from build123d import *

# Parameters (mm, degrees)
SKETCH2_R           = 1.7
BOSS_EXTRUDE1_DEPTH = 3.175
CUT_EXTRUDE1_DEPTH  = 4.175


with BuildPart() as part:
    # Sketch2 → Boss-Extrude1 (new body)
    with BuildSketch(Plane.XY):
        with BuildLine():
            Line((54.582717937, -59.58290593), (54.582717937, 171.394622999))
            ThreePointArc((54.582717937, 171.394622999), (24.582717937, 201.394622999), (-5.417282063, 171.394622999))
            Line((-5.417282063, 171.394622999), (-5.417282063, -59.58290593))
            ThreePointArc((-5.417282063, -59.58290593), (24.582717937, -89.58290593), (54.582717937, -59.58290593))
        make_face()
        with Locations((27.882717937, 197.940291196)):
            Circle(SKETCH2_R, mode=Mode.SUBTRACT)
        with Locations((-2.167282063, -59.58290593)):
            Circle(SKETCH2_R, mode=Mode.SUBTRACT)
        with Locations((5.667611541, -78.498012327)):
            Circle(SKETCH2_R, mode=Mode.SUBTRACT)
        with Locations((21.182717937, -86.115951364)):
            Circle(SKETCH2_R, mode=Mode.SUBTRACT)
        with Locations((51.332717937, 171.394622999)):
            Circle(SKETCH2_R, mode=Mode.SUBTRACT)
        with Locations((-2.167282063, 59.305858535)):
            Circle(SKETCH2_R, mode=Mode.SUBTRACT)
        with Locations((27.982717937, -86.115951364)):
            Circle(SKETCH2_R, mode=Mode.SUBTRACT)
        with Locations((-2.167282063, 171.394622999)):
            Circle(SKETCH2_R, mode=Mode.SUBTRACT)
        with Locations((51.332717937, 115.905858535)):
            Circle(SKETCH2_R, mode=Mode.SUBTRACT)
        with Locations((-2.167282063, 115.905858535)):
            Circle(SKETCH2_R, mode=Mode.SUBTRACT)
        with Locations((43.497824334, -78.498012327)):
            Circle(SKETCH2_R, mode=Mode.SUBTRACT)
        with Locations((51.332717937, -59.58290593)):
            Circle(SKETCH2_R, mode=Mode.SUBTRACT)
        with Locations((51.332717937, -34.094141465)):
            Circle(SKETCH2_R, mode=Mode.SUBTRACT)
        with Locations((-2.167282063, -34.094141465)):
            Circle(SKETCH2_R, mode=Mode.SUBTRACT)
        with Locations((51.332717937, -4.094141465)):
            Circle(SKETCH2_R, mode=Mode.SUBTRACT)
        with Locations((-2.167282063, -4.094141465)):
            Circle(SKETCH2_R, mode=Mode.SUBTRACT)
        with Locations((51.332717937, 25.905858535)):
            Circle(SKETCH2_R, mode=Mode.SUBTRACT)
        with Locations((-2.167282063, 25.905858535)):
            Circle(SKETCH2_R, mode=Mode.SUBTRACT)
        with Locations((21.282717937, 197.940291196)):
            Circle(SKETCH2_R, mode=Mode.SUBTRACT)
        with Locations((51.332717937, 52.505858535)):
            Circle(SKETCH2_R, mode=Mode.SUBTRACT)
        with Locations((51.332717937, 59.305858535)):
            Circle(SKETCH2_R, mode=Mode.SUBTRACT)
        with Locations((-2.167282063, 52.505858535)):
            Circle(SKETCH2_R, mode=Mode.SUBTRACT)
    extrude(amount=BOSS_EXTRUDE1_DEPTH)

    # Sketch3 → Cut-Extrude1 (cut, through all)
    with BuildSketch(Plane.XY.offset(3.175)):
        Polygon((-23.178598576, 28.330849589), (72.344034451, 83.480867481), (72.344034451, -133.046541286), (-23.178598576, -133.046541286), align=None)
    extrude(amount=-CUT_EXTRUDE1_DEPTH, mode=Mode.SUBTRACT)


solid = part.part
The model under review builds one solid part; all positions refer to its coordinate system, in mm. Coordinates: 2 decimals unless noted, no trailing zeros. Order: outer loops, then holes, each group sorted by start corner. A loop starts at its lowest first (then second) coordinate and runs counter-clockwise, first axis right, second up. Notation, with made-up numbers: (14.25, -33) -> (39.25, -33) arc R31 cw to (39.25, -3) -> close; hole circle Ø2 at (63, -7.5). An arc over 180 degrees is marked (long way). Answer in a Markdown table with one row per item.
(1) Consider section A-A (z = 2.2). State how many separate pieces and enclosed holes the cut face has, plus the area to 3 significant figures.
Answers:
| item | result |
|---|---|
| separate pieces | 1 |
| enclosed holes | 8 |
| area | 8,270 mm² |
(2) Consider section C-C (x = 4.5). Write out the cut boundary in (y, z) (3 decimals), plus the area to 3 significant figures.
Answers:
| item | result |
|---|---|
| outline | (44.311, 0) -> (193.681, 0) -> (193.681, 3.175) -> (44.311, 3.175) -> close |
| area | 474 mm² |
(3) Wall thickness on line 1 along Y through (x, z) = (50.5, 0.8); line 2 along X through (y, z) = (172, 0.1); line 3 along X through (y, z) = (58, 0.65): over which ranges is each line inside the solid? List them lowest first.
Answers:
| item | result |
|---|---|
| line 1 | 70.87 to 114.42, 117.39 to 169.91, 172.88 to 186.5 |
| line 2 | -5.41 to -3.76, -0.58 to 49.74, 52.92 to 54.58 |
| line 3 | -5.42 to -3.26, -1.08 to 28.21 |
(4) Consider section B-B (y = 178). Write out the cut boundary in (x, z) (1 decimal), plus the area to 3 significant figures.
Answers:
| item | result |
|---|---|
| outline | (-4.7, 0) -> (53.8, 0) -> (53.8, 3.2) -> (-4.7, 3.2) -> close |
| area | 186 mm² |
(5) Insertion check: pin 1 (4.5 mm diameter, centred on x = -2.17, y = 59.31, fed in from +Z) (3 decimals); pin 2 (2 mm diameter, centred on x = -2.17, y = 171.39, fed in from +Z). Each pin has a flat end and moves straight along its axis. Give the tip position at first contact, or say it passes through.
Answers:
| item | result |
|---|---|
| pin 1 | z = 3.175 |
| pin 2 | through |
(6) The part is to be moulded in two halves that separate along Y. For faces 1 (the flat face through (24, 121, 3.175)), 2 (the flat face through (24.16, 55.66, 1.61)), 3 (the cylindrical face through (-2.39, 173.08, 1.57)), 4 (the cylindrical face through (51.11, 173.08, 1.57)), say which applies: +Y half, -Y half, draft (parallel to the pull), parting line (faces both ways), or undercut.
Answers:
| item | result |
|---|---|
| face 1 | draft |
| face 2 | -Y half |
| face 3 | undercut |
| face 4 | undercut |
